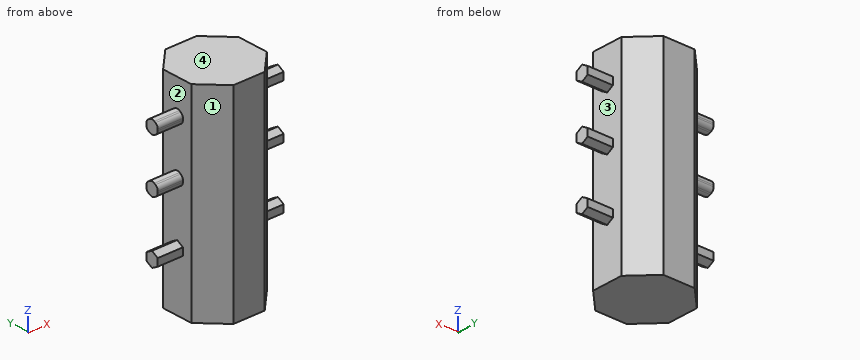
from build123d import *

# Parameters (mm, degrees)
F1_DEPTH      = 101.6
F3_DEPTH      = 12.7
F3_DEPTH_BACK = 50.8
F4_R          = 2.54
F5_R          = 2.54


with BuildPart() as f1:
    # F0 (on Top) → F1 (new body)
    with BuildSketch(Plane.XY):
        Polygon((19.05, -7.8907683632), (19.05, 7.8907683632), (7.8907683632, 19.05), (-7.8907683632, 19.05), (-19.05, 7.8907683632), (-19.05, -7.8907683632), (-7.8907683632, -19.05), (7.8907683632, -19.05), align=None)
    extrude(amount=F1_DEPTH)

    # F2 (on face) → F3 (join, two sides)
    with BuildSketch(Plane.YZ.offset(19.05)) as f3_sk:
        Polygon((3.175, 82.9758370032), (3.175, 86.6420112126), (0, 88.4750983173), (-3.175, 86.6420112126), (-3.175, 82.9758370032), (0, 81.1427498985), align=None)
        Polygon((3.175, 56.5934885845), (3.175, 60.2596627939), (0, 62.0927498985), (-3.175, 60.2596627939), (-3.175, 56.5934885845), (0, 54.7604014798), align=None)
        Polygon((3.175, 26.6308819025), (3.175, 30.2970561118), (0, 32.1301432165), (-3.175, 30.2970561118), (-3.175, 26.6308819025), (0, 24.7977947978), align=None)
    extrude(amount=F3_DEPTH)
    extrude(f3_sk.sketch, amount=-F3_DEPTH_BACK)

    # F4
    f4_edges = [f1.edges().sort_by_distance(p)[0] for p in [
        (-25.4, 3.175, 86.642011),
        (-25.4, 3.175, 82.975837),
        (-25.4, 0, 81.14275),
        (-25.4, -3.175, 82.975837),
        (-25.4, -3.175, 86.642011),
        (-25.4, 0, 88.475098),
    ]]
    fillet(f4_edges, radius=F4_R)

    # F5
    f5_edges = [f1.edges().sort_by_distance(p)[0] for p in [
        (-25.4, 0, 62.09275),
        (-25.4, -3.175, 56.593489),
        (-25.4, 0, 54.760401),
        (-25.4, 3.175, 56.593489),
        (-25.4, 3.175, 60.259663),
        (-25.4, -3.175, 60.259663),
    ]]
    fillet(f5_edges, radius=F5_R)


solid = f1.part
Could you check a few things on this model? Use its own coordinates, in mm. Face numbers are marked on the shaded views. Give positions to 0.01 mm unless a question says otherwise; leave off trailing zeros. Write each loop counter-clockwise with the first axis right and the second up, starting at its lowest first coordinate (ties: lowest second). Pieces come first, ordered by that corner, then holes. Notation, with made-up numbers: (-39.75, 20.5) - (-6.75, 20.5) arc R19 ccw to (-6.75, 31.5) - close; hole circle Ø6 at (18.25, 69.25). An arc over 180 degrees is marked (long way). Use CSV: the item, a comma, the result in double quotes. Start each with the question number.
Item 1: I want a section at A-A, the plane z = 73. Please give me the cut outline in (x, y), then the cut area to 3 significant figures.
Item 2: I want a section at C-C, the plane x = -15. Please give me the cut outline in (y, z).
Item 3: I'm going to push flat-ended pins straight in: pin 1 (1 mm diameter, centred on y = 11.5, z = 73.5, fed in from -X); pin 2 (5 mm diameter, centred on y = -6, z = 81.5, fed in from -X); pin 3 (1.1 mm diameter, centred on x = 25, z = 58, fed in from -Y) (3 decimals). Where does each tip first touch, or does it pass through?
Item 4: If I drill on line 1 along Z through (x, y) = (26, -2.5); line 2 along Z through (x, y) = (21.5, 3); line 3 along Y through (x, z) = (20.5, 84) (3 decimals), over which ranges is the centre line in solid material (lowest first)?
Item 5: If we mould it in two halves opening along Z, with no side actions, what happens to the marked faces 1, 2, 3 and 4? For each: pulls with the +Z half, pulls with the -Z half, needs draft (parallel to the pull), parting line crosses it, or undercut.
Item 6: I want a section at B-B, the plane y = -5. Please give me the cut outline in (x, z).
Findings:
1,outline,"(-19.05, -7.89) - (-7.89, -19.05) - (7.89, -19.05) - (19.05, -7.89) - (19.05, 7.89) - (7.89, 19.05) - (-7.89, 19.05) - (-19.05, 7.89) - close"
1,area,"1,200 mm2"
2,outline,"(-11.94, 0) - (11.94, 0) - (11.94, 101.6) - (-11.94, 101.6) - close"
3,pin 1,"stops at x = -15.94"
3,pin 2,"stops at x = -19.05"
3,pin 3,"stops at y = -3.175"
4,line 1,"z = 26.24 to 30.69, 56.2 to 60.65, 82.59 to 87.03"
4,line 2,"z = 26.53 to 30.4, 56.49 to 60.36, 82.87 to 86.74"
4,line 3,"y = -3.175 to 3.175"
5,face 1,"needs draft"
5,face 2,"undercut"
5,face 3,"undercut"
5,face 4,"pulls with the +Z half"
6,outline,"(-19.05, 0) - (19.05, 0) - (19.05, 101.6) - (-19.05, 101.6) - close"
